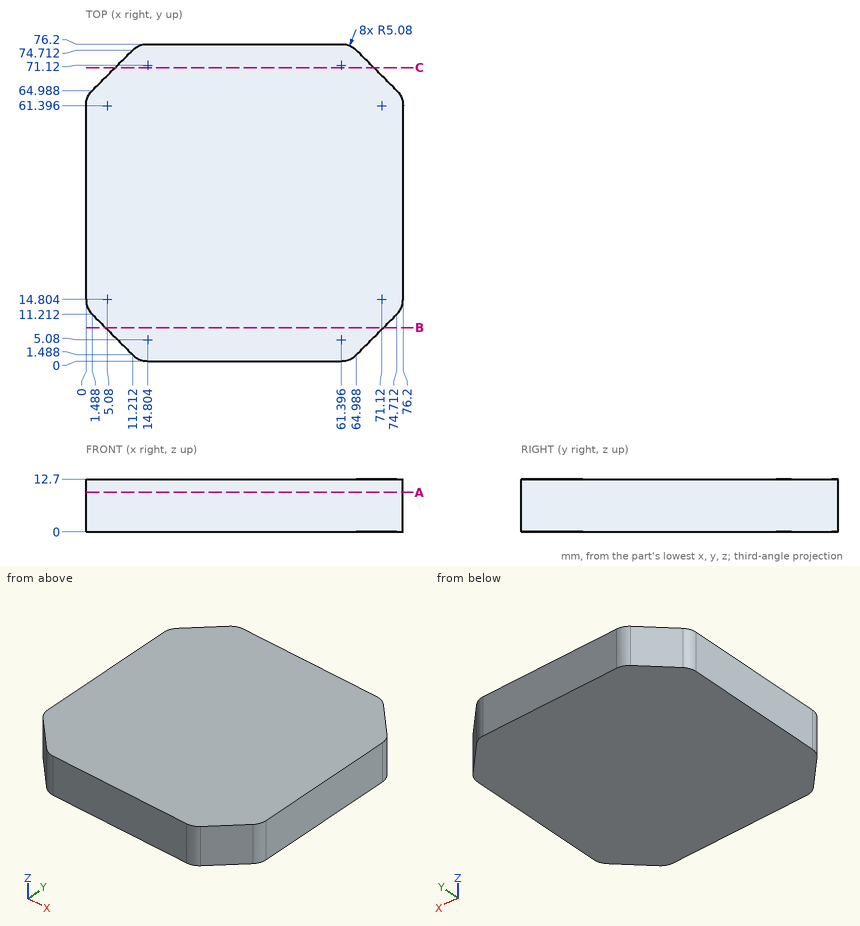
Answer from the drawing. Dimensions are ordinates in mm from the lowest x, y and z of the part. Coordinates: 2 decimals unless noted, no trailing zeros. Write each loop counter-clockwise with the first axis right and the second up, starting at its lowest first coordinate (ties: lowest second). Pieces come first, ordered by that corner, then holes. Notation, with made-up numbers: M 57.25,-25.5 L 84.25,-25.5 A16 cw 84.25,-21.5 Z; hole C 19.25,69 d9. An arc over 180 degrees is marked long. Put each result on its own line as item: value. Start each with the question number.
1. A cutting plane is placed at C-C on y = 70.5. Write down the section's boundary in (x, z), then the cut area to 3 significant figures.
2. Consider line 1 (Y direction, x = 6, z = 8.25); line 2 (X direction, y = 71, z = 8.5); line 3 (Y direction, x = 68, z = 11.5). Determine where each line is inside the solid, lowest interval first. Write a range as from..to.
3. A cutting plane is placed at A-A on z = 9.5. Write down the section's boundary in (x, y), then the cut area to 3 significant figures.
4. Flat-ended cylindrical pins translate along their axes: P1, Ø6, axis at x = 65.5, z = 9, coming from the -Y side; P2, Ø1.5, axis at y = 12.5, z = 11, coming from the +X side; P3, Ø8, axis at x = 68, y = 21.5, coming from the -Z side; P4, Ø1, axis at y = 13.5, z = 7.5, coming from the -X side. Find the tip coordinate at first contact, or state that the pin passes through.
5. A cutting plane is placed at B-B on y = 8. Write down the section's boundary in (x, z), then the cut area to 3 significant figures.
Resolved:
1. outline: M 7,0 L 69.2,0 L 69.2,12.7 L 7,12.7 Z
1. area: 790 mm2
2. line 1: y = 6.7..69.5
2. line 2: x = 7.5..68.7
2. line 3: y = 4.5..71.7
3. outline: M 0,14.8 A5.08 ccw 1.49,11.21 L 11.21,1.49 A5.08 ccw 14.8,0 L 61.4,0 A5.08 ccw 64.99,1.49 L 74.71,11.21 A5.08 ccw 76.2,14.8 L 76.2,61.4 A5.08 ccw 74.71,64.99 L 64.99,74.71 A5.08 ccw 61.4,76.2 L 14.8,76.2 A5.08 ccw 11.21,74.71 L 1.49,64.99 A5.08 ccw 0,61.4 Z
3. area: 5,480 mm2
4. P1: stops at y = 0.12
4. P2: stops at x = 75.96
4. P3: stops at z = 0
4. P4: stops at x = 0.06
5. outline: M 4.7,0 L 71.5,0 L 71.5,12.7 L 4.7,12.7 Z
5. area: 848 mm2
